Design review of the part built by this model. Coordinates are the model's own, in mm. A direction names the side the tool comes from. Give positions to 0.01 mm unless a question says otherwise; leave off trailing zeros. Write each loop counter-clockwise with the first axis right and the second up, starting at its lowest first coordinate (ties: lowest second). Pieces come first, ordered by that corner, then holes. Notation, with made-up numbers: (80.25, 62.5) -> (92.25, 62.5) arc R24 ccw to (92.25, 95.5) -> close; hole circle Ø8 at (-33, 57.25). An arc over 180 degrees is marked (long way). Write each question's results on one line, items separated by ' | '. Start each with the question number.
(1) Take a section at C-C (x = -1.5). State the section outline as (y, z) points, plus the area to 3 significant figures.
(2) Take a section at A-A (y = 2.5). State the section outline as (x, z) points.
(3) To check wall thickness, follow probe 1 along X at (y, z) = (5, 0); probe 2 along Z at (x, y) = (0, 7.5); probe 3 along Z at (x, y) = (-14, 2). State the ranges of each line that lie inside material, in increasing order.
(4) Take a section at B-B (y = 10.25). State the section outline as (x, z) points.
(5) For faces 1 (the face through (-1, 2, 5)), 2 (the face through (-19.458, 1.521, -6.233)), 3 (the face through (-1.08, 8.42, -4.88)), list the 3-axis set-ups (+Z, -Z, +X, -X, +Y, -Y) from which the entire face can be reached by the end or side of a thin tool; tool diameter is ignored.
(6) Take a section at D-D (x = 12.5). State the section outline as (y, z) points, plus the area to 3 significant figures.
(7) Clearance check with flat-ended pins moving along their axes: pin 1 (1.5 mm diameter, centred on x = 4.5, y = 1, fed in from -Z); pin 2 (3 mm diameter, centred on x = -8, z = 5, fed in from +Y); pin 3 (3.5 mm diameter, centred on x = 2, y = 1.5, fed in from +Z). State where each tip first meets the part, or that it passes through.
Autodesk Inventor part; units mm, degrees
ref_plane "YZ Plane" through (0, 0, 0) normal (1, 0, 0) x (0, 1, 0)
ref_plane "XZ Plane" through (0, 0, 0) normal (0, 1, 0) x (-1, 0, 0)
ref_plane "XY Plane" through (0, 0, 0) normal (0, 0, 1) x (1, 0, 0)
sketch "Sketch1" plane through (0, 0, 0) normal (0, 1, 0) x (-1, 0, 0)
  line L0 (22.5, -7.5) -> (22.5, 7.5)
  line L1 (22.5, 7.5) -> (-22.5, 7.5)
  line L2 (-22.5, -7.5) -> (22.5, -7.5)
  line L3 (-30, 0) -> (22.5, 0)
  line L4 (-22.5, -7.5) -> (-22.5, 7.5)
  line L5 (0, -7.5) -> (0, 7.5)
  line L6 (-22.5, -7.5) -> (-22.5, 7.5)
  point P0 (0, 0)
  dimension "d0" = 15
  dimension "d1" = 45
extrude "Extrusion1" add sketch "Sketch1" along normal blind 3
sketch "Sketch2" plane through (0, 3, 0) normal (0, 1, 0) x (1, 0, 0)
  circle A0 centre (0, 0) radius 5
  arc A1 (2.4, 1.9621) -> (2.4, -1.9621) centre (0, 0) ccw
  line L0 (2.4, 1.9621) -> (2.4, -1.9621)
  dimension "d4" = 10
  dimension "d5" = 3.1
  dimension "d6" = 2.4
extrude "Extrusion2" add sketch "Sketch2" along normal blind 11
sketch "Sketch3" plane through (0, 3, 0) normal (0, 1, 0) x (1, 0, 0)
  line L0 (22.5, -7.5) -> (22.5, 7.5)
  line L1 (22.5, 0) -> (14.5, 7.5)
  line L2 (22.5, 7.5) -> (-22.5, 7.5)
  line L3 (14.5, 7.5) -> (14.5, 5)
  line L4 (14.5, 5) -> (-16.5, 5)
  line L5 (-22.5, 7.5) -> (-22.5, -7.5)
  line L6 (-16.5, 5) -> (-22.5, 7.5)
  line L7 (-22.5, 7.5) -> (-22.5, -7.5)
  line L8 (-22.5, 0) -> (22.5, 0)
  line L9 (22.5, 0) -> (14.5, -7.5)
  line L10 (-22.5, -7.5) -> (22.5, -7.5)
  line L11 (14.5, -7.5) -> (14.5, -5)
  line L12 (14.5, -5) -> (-16.5, -5)
  line L13 (-16.5, -5) -> (-22.5, -7.5)
  point P0 (0, 0)
  dimension "d9" = 2.5
  dimension "d10" = 8
  dimension "d11" = 6
  dimension "d14" = 6
  dimension "d15" = 2.5
  dimension "d16" = 8
extrude "Extrusion3" cut sketch "Sketch3" against normal through all contours L10 L9 L0 | L1 L2 L0 | L10 L13 L12 L11 | L3 L4 L6 L2
properties part number "Motor_arrow_v02"
Report:
1) outline: (0, -5) -> (3, -5) -> (3, -4.77) -> (14, -4.77) -> (14, -2.71) -> (3, -2.71) -> (3, 2.71) -> (14, 2.71) -> (14, 4.77) -> (3, 4.77) -> (3, 5) -> (0, 5) -> close | area: 75.2 mm2
2) outline: (-22.5, -7.5) -> (-16.5, -5) -> (14.5, -5) -> (14.5, -7.5) -> (22.5, 0) -> (14.5, 7.5) -> (14.5, 5) -> (-16.5, 5) -> (-22.5, 7.5) -> close
3) probe 1: -5 to -3.1, 2.4 to 5 | probe 2: -5 to -3.1, 3.1 to 5 | probe 3: -5 to 5
4) outline: circle Ø10 at (0, 0); hole (2.4, -1.96) -> (2.4, 1.96) arc R3.1 ccw (long way) to start
5) face 1: +Z, +Y, -Y | face 2: -Z, +Y, -Y | face 3: +Y
6) outline: (0, -5) -> (3, -5) -> (3, 5) -> (0, 5) -> close | area: 30.0 mm2
7) pin 1: z = -5 | pin 2: y = 3 | pin 3: z = 5
